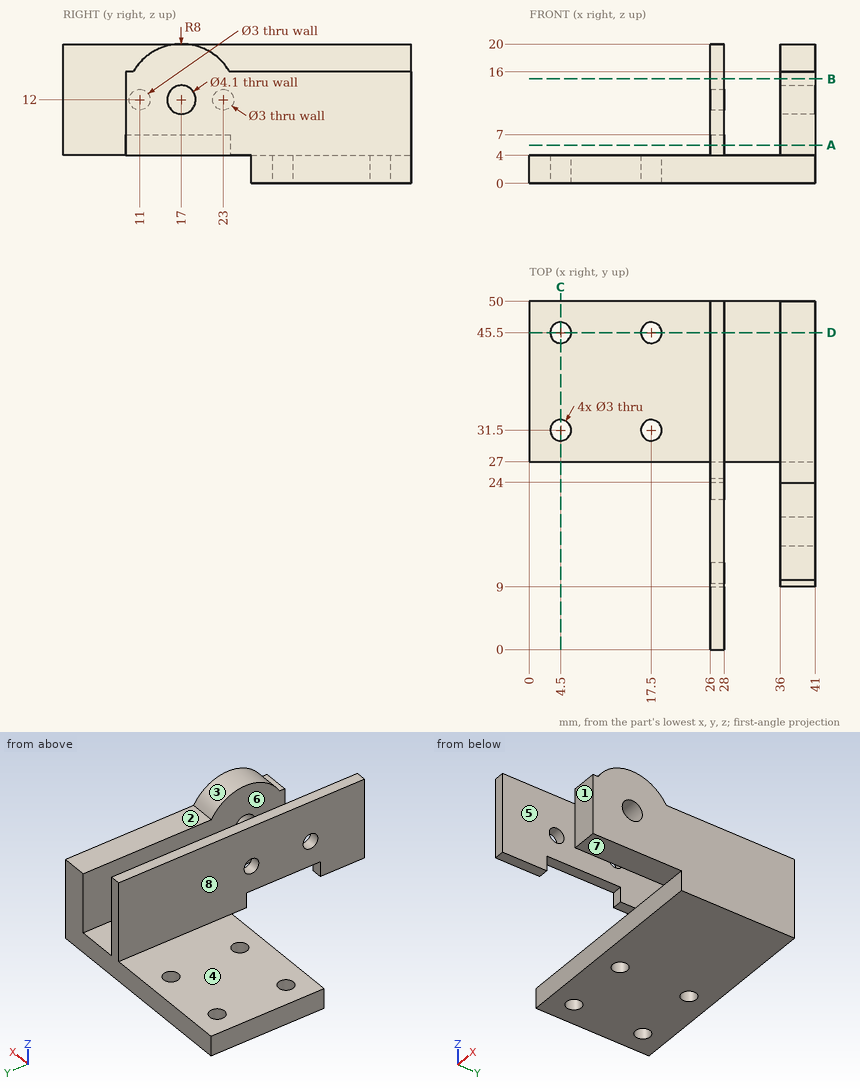
Drawing for the job (mm, zero at the part's lowest x, y, z). A direction names the side the tool comes from. Round coordinates to 2 decimals unless told otherwise and drop trailing zeros. Loops run counter-clockwise (first coordinate to the right, second up) from the corner with the lowest first, then second, coordinate; pieces in that order, holes last.
1. Wall check: probe 1 along Y at (x, z) = (17.5, 2.95); probe 2 along X at (y, z) = (45.5, 2.15); probe 3 along X at (y, z) = (36, 10.5). Give the ranges that are in metal, low to high.
Check values:
probe 1: y = 27 to 30, 33 to 44, 47 to 50
probe 2: x = 0 to 3, 6 to 16, 19 to 41
probe 3: x = 26 to 28, 36 to 41
2. Band-saw the part on B-B, the plane z = 15. List the corners of the cut face in (x, y), and give its area (3 significant figures).
Check values:
outline: (26, 0) - (28, 0) - (28, 50) - (26, 50) - close; (36, 9) - (41, 9) - (41, 50) - (36, 50) - close
area: 305 mm2
3. Tool access for the marked faces 1, 2, 3, 4 and 5: list every direction of +Z, -Z, +X, -X, +Y, -Y with a clear straight run to the whole face (end or side of a thin tool).
Check values:
face 1: +Z, -Z, +X, -Y
face 2: +Z, +X, +Y
face 3: +Z, +X
face 4: +Z, -X, +Y, -Y
face 5: +Z, +Y, -Y
4. Band-saw the part on D-D, the plane y = 45.5. List the corners of the cut face in (x, z).
Check values:
outline: (0, 0) - (3, 0) - (3, 4) - (0, 4) - close; (6, 0) - (16, 0) - (16, 4) - (6, 4) - close; (19, 0) - (41, 0) - (41, 16) - (36, 16) - (36, 4) - (28, 4) - (28, 20) - (26, 20) - (26, 4) - (19, 4) - close
5. Mould opens along X. For the marked faces 6, 7 and 8 say: +X half, -X half, draft (parallel to the pull), parting line (faces both ways), or undercut.
Check values:
face 6: undercut
face 7: draft
face 8: -X half
6. Band-saw the part on C-C, the plane x = 4.5. List the corners of the cut face in (y, z), and give its area (3 significant figures).
Check values:
outline: (27, 0) - (30, 0) - (30, 4) - (27, 4) - close; (33, 0) - (44, 0) - (44, 4) - (33, 4) - close; (47, 0) - (50, 0) - (50, 4) - (47, 4) - close
area: 68.0 mm2
7. Band-saw the part on A-A, the plane z = 5.5. List the corners of the cut face in (x, y).
Check values:
outline: (26, 0) - (28, 0) - (28, 9) - (26, 9) - close; (26, 24) - (28, 24) - (28, 50) - (26, 50) - close; (36, 9) - (41, 9) - (41, 50) - (36, 50) - close
8. Drop flat-ended pins along their axis: P1, Ø1.6, axis at x = 27.5, z = 6, coming from the -Y side; P2, Ø1.5, axis at x = 33.5, y = 14, coming from the -Z side; P3, Ø12, axis at x = 13.5, z = 9.5, coming from the -Y side; P4, Ø5, axis at y = 33.5, z = 11.5, coming from the -X side. Give the stop position or say it passes through.
Check values:
P1: stops at y = 0
P2: passes through
P3: stops at y = 27
P4: stops at x = 26
